Build history of the part. All positions in model axes, mm. Face numbers are marked on the shaded views. Give positions to 0.01 mm unless a question says otherwise; leave off trailing zeros. Order: outer loops, then holes, each group sorted by start corner. A loop starts at its lowest first (then second) coordinate and runs counter-clockwise, first axis right, second up. Notation, with made-up numbers: (37.5, -38) - (73.5, -38) arc R25 cw to (73.5, -14) - close; hole circle Ø4 at (-28.75, 88). An arc over 180 degrees is marked (long way). Use a Markdown table: item, result. Add a question column.
(1) Slice it at A-A (y = -49). Write the cut outline in (x, z), then the cut area to 3 significant figures.
(2) Wall check: line 1 (X direction, y = -39.6, z = -1.25); line 2 (X direction, y = -41.5, z = -7); line 3 (Z direction, x = -24, y = -50). Give the ranges that are in metal, low to high.
(3) Mould opens along X. For the marked faces 1, 2, 3 and 4 say: +X half, -X half, draft (parallel to the pull), parting line (faces both ways), or undercut.
(4) Slice it at B-B (x = -39.6). Write the cut outline in (y, z).
(5) Slice it at D-D (y = -40). Write the cut outline in (x, z), then the cut area to 3 significant figures.
(6) Flat gauge pins, fed straight in: pin 1 (2 mm diameter, centred on x = 40, y = -31, fed in from -Z); pin 2 (3 mm diameter, centred on x = -10.5, z = -4.5, fed in from +Y); pin 3 (2 mm diameter, centred on y = -46, z = -6, fed in from -X); pin 4 (2 mm diameter, centred on x = 24.5, y = -45.5, fed in from -Z). Where does each tip first touch, or does it go through?
(7) Slice it at C-C (z = -5). Write the cut outline in (x, y).
from build123d import *

# Parameters (mm, degrees)
CYLINDER1328_R               = 59
CYLINDER1328_DEPTH           = 40
CYLINDER1046_R               = 1.5
CYLINDER1046_DEPTH           = 20
CYLINDER1047_R               = 1.5
CYLINDER1047_DEPTH           = 20
CYLINDER1044_R               = 1.5
CYLINDER1044_DEPTH           = 20
CYLINDER1048_R               = 1.5
CYLINDER1048_DEPTH           = 20
BOX435_W                     = 6
BOX435_H                     = 2
BOX435_DEPTH                 = 6
BOX436_W                     = 6
BOX436_H                     = 2
BOX436_DEPTH                 = 6
BOX434_W                     = 6
BOX434_H                     = 2
BOX434_DEPTH                 = 6
BOX437_W                     = 6
BOX437_H                     = 2
BOX437_DEPTH                 = 6
CYLINDER1045_R               = 4
CYLINDER1045_DEPTH           = 20
CYLINDER1045_PLACEMENT_ANGLE = 45
CYLINDER1040_R               = 4
CYLINDER1040_DEPTH           = 20
CYLINDER1040_PLACEMENT_ANGLE = 45
CYLINDER1043_R               = 10
CYLINDER1043_DEPTH           = 40
CYLINDER1041_R               = 10
CYLINDER1041_DEPTH           = 40
CYLINDER1042_R               = 52
CYLINDER1042_DEPTH           = 8
BOX438_W                     = 108
BOX438_H                     = 36
BOX438_DEPTH                 = 8
FILLET016_R                  = 12


with BuildPart() as obj1:
    # Cylinder1328 → Cylinder1328 (new body)
    with BuildSketch(Plane(origin=(0, -17, 21), x_dir=(1, 0, 0), z_dir=(0, -1, 0))):
        Circle(CYLINDER1328_R)
    extrude(amount=CYLINDER1328_DEPTH)


with BuildPart() as obj2:
    # Cylinder1046 → Cylinder1046 (new body)
    with BuildSketch(Plane(origin=(24, -40, -5), x_dir=(1, 0, 0), z_dir=(0, -1, 0))):
        Circle(CYLINDER1046_R)
    extrude(amount=CYLINDER1046_DEPTH)


with BuildPart() as obj3:
    # Cylinder1047 → Cylinder1047 (new body)
    with BuildSketch(Plane(origin=(51, -40, 7), x_dir=(1, 0, 0), z_dir=(0, -1, 0))):
        Circle(CYLINDER1047_R)
    extrude(amount=CYLINDER1047_DEPTH)


with BuildPart() as obj4:
    # Cylinder1044 → Cylinder1044 (new body)
    with BuildSketch(Plane(origin=(-51, -40, 7), x_dir=(1, 0, 0), z_dir=(0, -1, 0))):
        Circle(CYLINDER1044_R)
    extrude(amount=CYLINDER1044_DEPTH)


with BuildPart() as compound827:
    # Cylinder1048 → Cylinder1048 (new body)
    with BuildSketch(Plane(origin=(-24, -40, -5), x_dir=(1, 0, 0), z_dir=(0, -1, 0))):
        Circle(CYLINDER1048_R)
    extrude(amount=CYLINDER1048_DEPTH)

    # Compound827: union obj2, obj3, obj4
    add(obj2.part)
    add(obj3.part)
    add(obj4.part)


with BuildPart() as krychle435:
    # Box435 → Box435 (new body)
    with BuildSketch(Plane(origin=(21, -47, -8), x_dir=(1, 0, 0), z_dir=(0, 0, 1))):
        with Locations((3, 1)):
            Rectangle(BOX435_W, BOX435_H)
    extrude(amount=BOX435_DEPTH)


with BuildPart() as krychle436:
    # Box436 → Box436 (new body)
    with BuildSketch(Plane(origin=(48, -45, 4), x_dir=(1, 0, 0), z_dir=(0, 0, 1))):
        with Locations((3, 1)):
            Rectangle(BOX436_W, BOX436_H)
    extrude(amount=BOX436_DEPTH)


with BuildPart() as krychle434:
    # Box434 → Box434 (new body)
    with BuildSketch(Plane(origin=(-54, -45, 4), x_dir=(1, 0, 0), z_dir=(0, 0, 1))):
        with Locations((3, 1)):
            Rectangle(BOX434_W, BOX434_H)
    extrude(amount=BOX434_DEPTH)


with BuildPart() as compound826:
    # Box437 → Box437 (new body)
    with BuildSketch(Plane(origin=(-27, -47, -8), x_dir=(1, 0, 0), z_dir=(0, 0, 1))):
        with Locations((3, 1)):
            Rectangle(BOX437_W, BOX437_H)
    extrude(amount=BOX437_DEPTH)

    # Compound826: union Krychle435, Krychle436, Krychle434
    add(krychle435.part)
    add(krychle436.part)
    add(krychle434.part)


with BuildPart() as obj5:
    # Cylinder1045 → Cylinder1045 (new body)
    with BuildSketch(Plane.XY):
        Circle(CYLINDER1045_R)
    extrude(amount=CYLINDER1045_DEPTH)


with BuildPart() as obj5_1:
    # Cylinder1045 placement: moved
    add(obj5.part.moved(Location((39.6, -39.6, -10))).rotate(Axis((39.6, -39.6, -10), (0, 0, 1)), CYLINDER1045_PLACEMENT_ANGLE))


with BuildPart() as compound829:
    # Cylinder1040 → Cylinder1040 (new body)
    with BuildSketch(Plane.XY):
        Circle(CYLINDER1040_R)
    extrude(amount=CYLINDER1040_DEPTH)


with BuildPart() as compound829_1:
    # Cylinder1040 placement: moved
    add(compound829.part.moved(Location((-39.6, -39.6, -10))).rotate(Axis((-39.6, -39.6, -10), (0, 0, -1)), CYLINDER1040_PLACEMENT_ANGLE))

    # Compound829: union obj5
    add(obj5_1.part)


with BuildPart() as obj6:
    # Cylinder1043 → Cylinder1043 (new body)
    with BuildSketch(Plane(origin=(-59, -17, 0), x_dir=(1, 0, 0), z_dir=(0, 0, 1))):
        Circle(CYLINDER1043_R)
    extrude(amount=CYLINDER1043_DEPTH)


with BuildPart() as compound828:
    # Cylinder1041 → Cylinder1041 (new body)
    with BuildSketch(Plane(origin=(59, -17, 0), x_dir=(1, 0, 0), z_dir=(0, 0, 1))):
        Circle(CYLINDER1041_R)
    extrude(amount=CYLINDER1041_DEPTH)

    # Compound828: union obj6
    add(obj6.part)


with BuildPart() as obj7:
    # Cylinder1042 → Cylinder1042 (new body)
    with BuildSketch(Plane.XY.offset(20)):
        Circle(CYLINDER1042_R)
    extrude(amount=CYLINDER1042_DEPTH)


with BuildPart() as common003:
    # Box438 → Box438 (new body)
    with BuildSketch(Plane(origin=(-54, -53, 20), x_dir=(1, 0, 0), z_dir=(0, 0, 1))):
        with Locations((54, 18)):
            Rectangle(BOX438_W, BOX438_H)
    extrude(amount=BOX438_DEPTH)

    # Cut435: cut obj7
    add(obj7.part, mode=Mode.SUBTRACT)


with BuildPart() as common003_1:
    # Cut435 placement: moved
    add(common003.part.moved(Location((0, 0, -20))))

    # Cut438: cut Compound828
    add(compound828.part, mode=Mode.SUBTRACT)


with BuildPart() as common003_2:
    # Cut438 placement: moved
    add(common003_1.part.moved(Location((0, 0, -8))))

    # Cut436: cut Compound829
    add(compound829_1.part, mode=Mode.SUBTRACT)

    # Cut437: cut Compound826
    add(compound826.part, mode=Mode.SUBTRACT)

    # Cut434: cut Compound827
    add(compound827.part, mode=Mode.SUBTRACT)

    # Fillet016
    fillet016_edges = [common003_2.edges().sort_by_distance(p)[0] for p in [
        (-54, -25.660254, -4),
        (54, -25.660254, -4),
    ]]
    fillet(fillet016_edges, radius=FILLET016_R)

    # Common003: intersect obj1
    add(obj1.part, mode=Mode.INTERSECT)


solid = common003_2.part
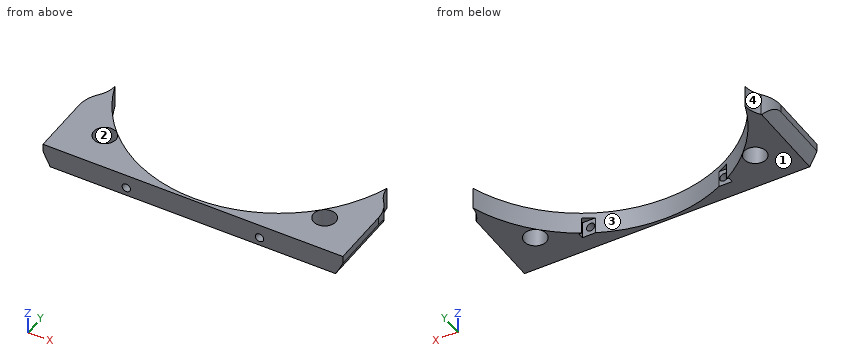
Solution:
| question | item | result |
|---|---|---|
| 1 | outline | (-54, -2.77) arc R59 ccw to (-51.38, -8) - (-17.41, -8) - (-17.41, 0) - (-54, 0) - close; (17.41, -8) - (51.38, -8) arc R59 ccw to (54, -2.77) - (54, 0) - (17.41, 0) - close; hole circle Ø3 at (-24, -5); hole circle Ø3 at (24, -5) |
| 1 | area | 558 mm2 |
| 2 | line 1 | -54 to -43.6, -35.6 to -33.7, 33.7 to 35.6, 43.6 to 54 |
| 2 | line 2 | -51.93 to -43.12, -36.08 to -31.33, 31.33 to 36.08, 43.12 to 51.93 |
| 2 | line 3 | -8 to -6.5, -3.5 to 0 |
| 3 | face 1 | draft |
| 3 | face 2 | undercut |
| 3 | face 3 | undercut |
| 3 | face 4 | -X half |
| 4 | outline | (-53, -8) - (-43.6, -8) - (-43.6, 0) - (-53, 0) - close; (-35.6, -8) - (-33.7, -8) - (-33.7, 0) - (-35.6, 0) - close |
| 5 | outline | (-54, -2.77) arc R59 ccw to (-51.38, -8) - (-43.58, -8) - (-43.58, 0) - (-54, 0) - close; (-35.62, -8) - (-33.23, -8) - (-33.23, 0) - (-35.62, 0) - close; (33.23, -8) - (35.62, -8) - (35.62, 0) - (33.23, 0) - close; (43.58, -8) - (51.38, -8) arc R59 ccw to (54, -2.77) - (54, 0) - (43.58, 0) - close |
| 5 | area | 192 mm2 |
| 6 | pin 1 | through |
| 6 | pin 2 | y = -50.6 |
| 6 | pin 3 | x = -52.96 |
| 6 | pin 4 | z = -2 |
| 7 | outline | (-52.96, -53) - (-25.5, -53) - (-25.5, -47) - (-27, -47) - (-27, -45) - (-26.06, -45) arc R52 cw to (-49.01, -17.39) arc R10 cw to (-51.27, -23.35) arc R12 ccw to (-52.96, -26.08) - close; (-22.5, -53) - (22.5, -53) - (22.5, -47) - (22.25, -47) arc R52 cw to (-22.25, -47) - (-22.5, -47) - close; (25.5, -53) - (52.96, -53) - (52.96, -26.08) arc R12 ccw to (51.27, -23.35) arc R10 cw to (49.01, -17.39) arc R52 cw to (26.06, -45) - (27, -45) - (27, -47) - (25.5, -47) - close; hole circle Ø8 at (-39.6, -39.6); hole circle Ø8 at (39.6, -39.6) |
